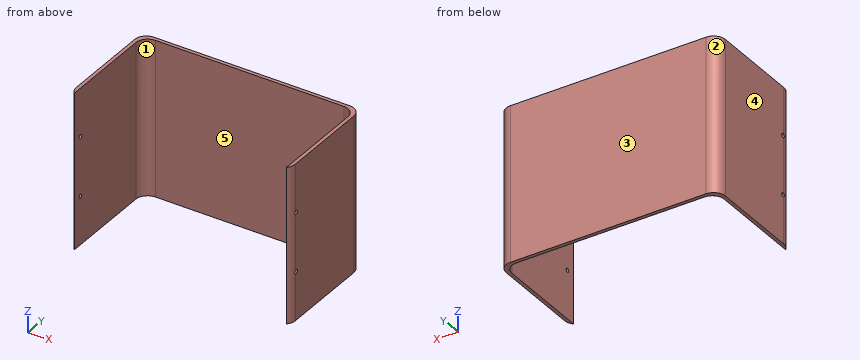
```python
from build123d import *

# Parameters (mm, degrees)
SKETCH1_W               = 132
SKETCH1_H               = 93
BOSS_EXTRUDE1_DEPTH     = 3
SKETCH3_W               = 132
SKETCH3_H               = 3
BOSS_EXTRUDE2_DEPTH     = 180
BOSS_EXTRUDE3_START     = 180
SKETCH4_W               = 132
SKETCH4_H               = 93
BOSS_EXTRUDE3_DEPTH     = 3
FILLET1_R               = 10
FILLET2_R               = 10
CUT_EXTRUDE1_DEPTH      = 245.053272873
CUT_EXTRUDE1_DEPTH_BACK = 245.053272873
SKETCH5_R               = 1.7


with BuildPart() as part:
    # Sketch1 → Boss-Extrude1 (new body)
    with BuildSketch(Plane(origin=(0, 0, 0), x_dir=(0, 0, -1), z_dir=(1, 0, 0))):
        with Locations((66, -46.5)):
            Rectangle(SKETCH1_W, SKETCH1_H)
    extrude(amount=BOSS_EXTRUDE1_DEPTH)

    # Sketch3 → Boss-Extrude2 (add)
    with BuildSketch(Plane.ZY):
        with Locations((-66, -1.5)):
            Rectangle(SKETCH3_W, SKETCH3_H)
    extrude(amount=BOSS_EXTRUDE2_DEPTH)

    # Sketch4 → Boss-Extrude3 (add)
    with BuildSketch(Plane.ZY.offset(BOSS_EXTRUDE3_START)):
        with Locations((-66, -46.5)):
            Rectangle(SKETCH4_W, SKETCH4_H)
    extrude(amount=BOSS_EXTRUDE3_DEPTH)

    # Fillet1
    fillet1_edges = [part.edges().sort_by_distance(p)[0] for p in [
        (0, -3, -66),
        (3, 0, -66),
        (-180, -3, -66),
        (-183, 0, -66),
    ]]
    fillet(fillet1_edges, radius=FILLET1_R)

    # Fillet2
    # the kernel refuses this fillet: 10 mm, written as the material it takes off along each edge
    with BuildSketch(Plane(origin=(3, -93, -149.853571071), x_dir=(0, 1, 0), z_dir=(0, 0, 1)), Plane(origin=(-183, -93, 17.853571071), x_dir=(0, 1, 0), z_dir=(0, 0, -1))) as fillet2_piece_1:
        with BuildLine():
            CenterArc((7.141428429, 10), FILLET2_R, 224.427004001, 45.572995999)
            Line((0, 3), (-0.142828569, 2.86))
            ThreePointArc((-0.142828569, 2.86), (-0.2, 1.5), (-0.2, 0))
            Line((-0.2, 0), (0, -0.2))
            Line((0, -0.2), (7.141428429, -0.2))
            Line((7.141428429, -0.2), (7.141428429, 0))
        make_face()
    extrude(amount=167.707142143, mode=Mode.SUBTRACT)

    # Sketch5 → Cut-Extrude1 (cut, two sides: drawn at the far end of the back side and taken through both)
    with BuildSketch(Plane.ZY.offset(-CUT_EXTRUDE1_DEPTH_BACK)):
        with Locations((-91, -85)):
            Circle(SKETCH5_R)
        with Locations((-41, -85)):
            Circle(SKETCH5_R)
    extrude(amount=CUT_EXTRUDE1_DEPTH + CUT_EXTRUDE1_DEPTH_BACK, mode=Mode.SUBTRACT)


solid = part.part
```
For this review, take the finished solid that the model builds, in its own axes (mm). Face numbers are marked on the shaded views. A direction names the side the tool comes from. Round coordinates to 2 decimals unless told otherwise and drop trailing zeros. Write each loop counter-clockwise with the first axis right and the second up, starting at its lowest first coordinate (ties: lowest second). Pieces come first, ordered by that corner, then holes. Notation, with made-up numbers: (58.5, 14.5) -> (82.5, 14.5) arc R30 cw to (82.5, 44.5) -> close; hole circle Ø1 at (47.25, 32). An arc over 180 degrees is marked (long way). One line per question, with ' | ' between items. Start each with the question number.
1) Mouldability with a two-part tool opening along X and no side actions: class the marked faces 3, 4 and 5 as +X half, -X half, draft (parallel to the pull), parting line (faces both ways), or undercut.
2) Wall thickness on line 1 along Z through (x, y) = (-181.35, -85); line 2 along X through (y, z) = (-52.5, -93); line 3 along Y through (x, z) = (-102, -125.5): over which ranges is each line inside the solid? List them lowest first.
3) Add section A-A (y = -69). Write out the cut boundary in (x, z), and give its area (3 significant figures).
4) For pin 1 Ø6 at (x, z) = (-109.5, -13.5) entering from -Y; pin 2 Ø4.5 at (y, z) = (-85, -41) entering from -X, all flat-tipped, find the tip position at first contact; note any pin that passes through.
5) Add section C-C (x = -146). Write out the cut boundary in (y, z), and give its area (3 significant figures).
6) Add section B-B (z = -71.5). Write out the cut boundary in (x, y), and give its area (3 significant figures).
7) Machinability: for the marked faces 1 and 2, which of the approach directions +Z, -Z, +X, -X, +Y, -Y give a long, thin tool a straight path to every point of the face, cutting with its end or side? Answer none if there is none.
Reported:
1) face 3: draft | face 4: -X half | face 5: undercut
2) line 1: z = -132 to -92.7, -89.3 to -42.7, -39.3 to 0 | line 2: x = -183 to -180, 0 to 3 | line 3: y = -3 to 0
3) outline: (-183, -132) -> (-180, -132) -> (-180, 0) -> (-183, 0) -> close; (0, -132) -> (3, -132) -> (3, 0) -> (0, 0) -> close | area: 792 mm²
4) pin 1: stops at y = -3 | pin 2: stops at x = -183
5) outline: (-3, -132) -> (0, -132) -> (0, 0) -> (-3, 0) -> close | area: 396 mm²
6) outline: (-183, -85.86) arc R10 ccw to (-180, -93) -> (-180, -13) arc R10 cw to (-170, -3) -> (-10, -3) arc R10 cw to (0, -13) -> (0, -93) arc R10 ccw to (3, -85.86) -> (3, -10) arc R10 ccw to (-7, 0) -> (-173, 0) arc R10 ccw to (-183, -10) -> close | area: 1,080 mm²
7) face 1: +Z, -Z, -Y | face 2: +Z, -Z, -X, +Y
